from build123d import *

# Parameters (mm, degrees)
SKETCH1_R           = 50
SKETCH1_R_2         = 5
BOSS_EXTRUDE1_DEPTH = 25
CUT_EXTRUDE1_START  = -5
SKETCH3_R           = 40
CUT_EXTRUDE1_DEPTH  = 20
CUT_EXTRUDE2_START  = 5
SKETCH3_2_R         = 40
CUT_EXTRUDE2_DEPTH  = 20


with BuildPart() as part:
    # Sketch1 → Boss-Extrude1 (new body, symmetric)
    with BuildSketch(Plane(origin=(0, 0, 0), x_dir=(0, 0, -1), z_dir=(1, 0, 0))):
        Circle(SKETCH1_R)
        Circle(SKETCH1_R_2, mode=Mode.SUBTRACT)
    extrude(amount=BOSS_EXTRUDE1_DEPTH, both=True)

    # Sketch3 → Cut-Extrude1 (cut)
    with BuildSketch(Plane(origin=(0, 0, 0), x_dir=(0, 0, -1), z_dir=(1, 0, 0)).offset(CUT_EXTRUDE1_START)):
        Circle(SKETCH3_R)
    extrude(amount=-CUT_EXTRUDE1_DEPTH, mode=Mode.SUBTRACT)

    # Sketch3_2 → Cut-Extrude2 (cut)
    with BuildSketch(Plane(origin=(0, 0, 0), x_dir=(0, 0, -1), z_dir=(1, 0, 0)).offset(CUT_EXTRUDE2_START)):
        Circle(SKETCH3_2_R)
    extrude(amount=CUT_EXTRUDE2_DEPTH, mode=Mode.SUBTRACT)


solid = part.part
Read the model definition and answer for the solid it produces. Units are mm, in the model's axes. A direction names the side the tool comes from. Coordinates: 2 decimals unless noted, no trailing zeros. Order: outer loops, then holes, each group sorted by start corner. A loop starts at its lowest first (then second) coordinate and runs counter-clockwise, first axis right, second up. Notation, with made-up numbers: (56, 57.25) -> (115, 57.25) arc R13 ccw to (115, 69.25) -> close; hole circle Ø6 at (16.5, 31). An arc over 180 degrees is marked (long way). Answer as a JSON object with one key per item and string values.
1) Each of these flat-tipped pins is pushed along its axis until it touches: pin 1 (3 mm diameter, centred on x = 3, y = -13, fed in from +Z); pin 2 (1 mm diameter, centred on y = 27.5, z = 3, fed in from +X); pin 3 (10 mm diameter, centred on x = -0.5, y = 34, fed in from +Z); pin 4 (9 mm diameter, centred on y = 0, z = 0, fed in from +X). Where does it stop, or does it pass through?
Model answer:
{"pin 1": "stops at z = 48.66", "pin 2": "stops at x = 5", "pin 3": "stops at z = 40.73", "pin 4": "passes through"}
2) The mould has two halves that part along Z. Classify faces 1 (the face through (5, 1, -8)), 2 (the face through (-25, 34, 22)), 3 (the face through (14.86, -39.05, 8.67)), 4 (the face through (0.35, 15.02, -47.69)): released by +Z, released by -Z, zero draft, split by the parting line, or undercut.
Model answer:
{"face 1": "undercut", "face 2": "zero draft", "face 3": "undercut", "face 4": "split by the parting line"}
3) Consider line 1 along Y through (x, z) = (-20, 0); line 2 along X through (y, z) = (-31, 22); line 3 along Z through (x, y) = (-14, -30.5). Determine where each line is inside the solid, lowest interval first. Write a range as from..to.
Model answer:
{"line 1": "y = -50..-40, 40..50", "line 2": "x = -5..5", "line 3": "z = -39.62..-25.88, 25.88..39.62"}
4) A cutting plane is placed at D-D, the plane y = 35. Determine the outline of the cut face in (x, z).
Model answer:
{"outline": "(-25, -35.71) -> (25, -35.71) -> (25, -19.36) -> (5, -19.36) -> (5, 19.36) -> (25, 19.36) -> (25, 35.71) -> (-25, 35.71) -> (-25, 19.36) -> (-5, 19.36) -> (-5, -19.36) -> (-25, -19.36) -> close"}
5) A cutting plane is placed at C-C, the plane x = 2. Determine the outline of the cut face in (y, z), plus the area to 3 significant figures.
Model answer:
{"outline": "circle Ø100 at (0, 0); hole circle Ø10 at (0, 0)", "area": "7,780 mm²"}
6) A tool of negligible diameter and unlimited length cuts with its end or side. For faces 5 (the face through (-14.86, -39.05, 8.67)), 6 (the face through (25, 34, 22)), from which of +Z, -Z, +X, -X, +Y, -Y can it reach the whole face along a straight path? Write none if from no direction.
Model answer:
{"face 5": "-X", "face 6": "+Z, -Z, +X, +Y, -Y"}
7) A cutting plane is placed at A-A, the plane z = 0. Determine the outline of the cut face in (x, y), plus the area to 3 significant figures.
Model answer:
{"outline": "(-25, -50) -> (25, -50) -> (25, -40) -> (5, -40) -> (5, -5) -> (-5, -5) -> (-5, -40) -> (-25, -40) -> close; (-25, 40) -> (-5, 40) -> (-5, 5) -> (5, 5) -> (5, 40) -> (25, 40) -> (25, 50) -> (-25, 50) -> close", "area": "1,700 mm²"}
